Build history of the part. All positions in model axes, mm. A direction names the side the tool comes from. Give positions to 0.01 mm unless a question says otherwise; leave off trailing zeros. Write each loop counter-clockwise with the first axis right and the second up, starting at its lowest first coordinate (ties: lowest second). Pieces come first, ordered by that corner, then holes. Notation, with made-up numbers: (38.5, 76) -> (55.5, 76) arc R31 ccw to (55.5, 104) -> close; hole circle Ø11 at (82, -28.5). An arc over 180 degrees is marked (long way). Put each result on its own line as item: value.
from build123d import *

# Parameters (mm, degrees)
SKETCH1_W               = 76
SKETCH1_H               = 40
BOSS_EXTRUDE1_DEPTH     = 6
BOSS_EXTRUDE2_START     = -10
BOSS_EXTRUDE2_OUTLINE_R = 6.5
BOSS_EXTRUDE2_DEPTH     = 10
SKETCH3_R               = 16
SKETCH3_R_2             = 6.5
BOSS_EXTRUDE3_DEPTH     = 4
SKETCH4_W               = 10
SKETCH4_H               = 41
BOSS_EXTRUDE4_DEPTH     = 30
CUT_EXTRUDE1_DEPTH      = 30
FILLET1_R               = 13
SKETCH6_R               = 6.5
CUT_EXTRUDE2_DEPTH      = 30


# Read off the part's stored shape, not the designer's step: Boss-Extrude2
with BuildPart() as part:
    # Sketch1 → Boss-Extrude1 (new body)
    with BuildSketch(Plane(origin=(0, 0, 0), x_dir=(1, 0, 0), z_dir=(0, 1, 0))):
        Rectangle(SKETCH1_W, SKETCH1_H)
    extrude(amount=-BOSS_EXTRUDE1_DEPTH)

    # Boss-Extrude2 outline → Boss-Extrude2 (add)
    with BuildSketch(Plane.XY.offset(20).offset(BOSS_EXTRUDE2_START)):
        with BuildLine():
            ThreePointArc((-16, 8), (-18.343145751, 2.343145751), (-24, 0))
            Line((-24, 0), (24, 0))
            ThreePointArc((24, 0), (18.343145751, 2.343145751), (16, 8))
            Line((16, 8), (16, 58))
            ThreePointArc((16, 58), (0, 74), (-16, 58))
            Line((-16, 58), (-16, 8))
        make_face()
        with Locations((0, 58)):
            Circle(BOSS_EXTRUDE2_OUTLINE_R, mode=Mode.SUBTRACT)
    extrude(amount=BOSS_EXTRUDE2_DEPTH)

    # Sketch3 → Boss-Extrude3 (add)
    with BuildSketch(Plane.XY.offset(20)):
        with Locations((0, 58)):
            Circle(SKETCH3_R)
        with Locations((0, 58)):
            Circle(SKETCH3_R_2, mode=Mode.SUBTRACT)
    extrude(amount=BOSS_EXTRUDE3_DEPTH)

    # Sketch4 → Boss-Extrude4 (add)
    with BuildSketch(Plane(origin=(0, 0, 10), x_dir=(-1, 0, 0), z_dir=(0, 0, -1))):
        with Locations((0, 20.5)):
            Rectangle(SKETCH4_W, SKETCH4_H)
    extrude(amount=BOSS_EXTRUDE4_DEPTH)

    # Sketch5 → Cut-Extrude1 (cut)
    with BuildSketch(Plane.ZY.offset(5)):
        Polygon((-20, 0), (10, 41), (-20, 41), align=None)
    extrude(amount=-CUT_EXTRUDE1_DEPTH, mode=Mode.SUBTRACT)

    # Fillet1
    fillet1_edges = [part.edges().sort_by_distance(p)[0] for p in [
        (-38, -3, -20),
        (38, -3, -20),
    ]]
    fillet(fillet1_edges, radius=FILLET1_R)

    # Sketch6 → Cut-Extrude2 (cut)
    with BuildSketch(Plane(origin=(0, 0, 0), x_dir=(1, 0, 0), z_dir=(0, 1, 0))):
        with Locations(Location((25, 7, 0), (0, 0, 270))):
            Circle(SKETCH6_R)
        with Locations(Location((-25, 7, 0), (0, 0, 270))):
            Circle(SKETCH6_R)
    extrude(amount=-CUT_EXTRUDE2_DEPTH, mode=Mode.SUBTRACT)


solid = part.part
1) Slice it at A-A (x = 0). Write the cut outline in (y, z), plus the area to 3 significant figures.
Filled sheet:
outline: (-6, -20) -> (0, -20) -> (41, 10) -> (51.5, 10) -> (51.5, 24) -> (42, 24) -> (42, 20) -> (-6, 20) -> close; (64.5, 10) -> (74, 10) -> (74, 24) -> (64.5, 24) -> close
area: 1,540 mm2
2) Slice it at C-C (y = 55). Write the cut outline in (x, z).
Filled sheet:
outline: (-16, 10) -> (-5.77, 10) -> (-5.77, 24) -> (-15.72, 24) -> (-15.72, 20) -> (-16, 20) -> close; (5.77, 10) -> (16, 10) -> (16, 20) -> (15.72, 20) -> (15.72, 24) -> (5.77, 24) -> close
3) Wall check: L1, parallel to X at y = -2, z = -10.5; L2, parallel to Z at x = 13, y = 44.5; L3, parallel to X at y = 20.5, z = 1. Give the ranges that are in metal, low to high.
Filled sheet:
L1: -37.52 to -30.48, -19.52 to 19.52, 30.48 to 37.52
L2: 10 to 20
L3: -5 to 5
4) Pin check, flat tips, straight feed: pin 1 (10 mm diameter, centred on y = 48.5, z = 10.5, fed in from -X); pin 2 (1.5 mm diameter, centred on x = -11, z = 5, fed in from +Y); pin 3 (6 mm diameter, centred on x = -4, y = 25.5, fed in from -Z); pin 4 (11.5 mm diameter, centred on x = 0, y = 58, fed in from +Z). Stop position of each tip, or through.
Filled sheet:
pin 1: x = -16
pin 2: y = 0
pin 3: z = -3.54
pin 4: through
5) Pull direction Z, two halves, no side cores. Call faces 1 (the cylindrical face through (18.406, 2.281, 14.93)), 2 (the cylindrical face through (-34.293, -3.042, -16.091)), 3 (the cylindrical face through (-19.519, -2.958, -3.506)): released by +Z, released by -Z, zero draft, split by the parting line, or undercut.
Filled sheet:
face 1: zero draft
face 2: released by -Z
face 3: undercut
6) Tool access for faces 4 (the flat face through (-6, 38, 10)), 5 (the flat face through (-16, 33, 15)), 6 (the flat face through (-5, 16, -1)), 7 (the cylindrical face through (-2.083, 73.864, 18.458)), 8 (the flat face through (21, 0, 0)): list every direction of +Z, -Z, +X, -X, +Y, -Y with a clear straight run to the whole face (end or side of a thin tool).
Filled sheet:
face 4: -Z, +Y
face 5: +Z, -Z, -X, +Y
face 6: -Z, -X, +Y
face 7: +Z
face 8: -Z, +X, +Y
7) Slice it at B-B (z = 14). Write the cut outline in (x, y).
Filled sheet:
outline: (-38, -6) -> (38, -6) -> (38, 0) -> (24, 0) arc R8 cw to (16, 8) -> (16, 58) arc R16 ccw to (-16, 58) -> (-16, 8) arc R8 cw to (-24, 0) -> (-38, 0) -> close; hole circle Ø13 at (0, 58)
8) Slice it at D-D (x = -26). Write the cut outline in (y, z), plus the area to 3 significant figures.
Filled sheet:
outline: (-6, -19.96) -> (0, -19.96) -> (0, -13.42) -> (-6, -13.42) -> close; (-6, -0.58) -> (0, -0.58) -> (0, 20) -> (-6, 20) -> close
area: 163 mm2
